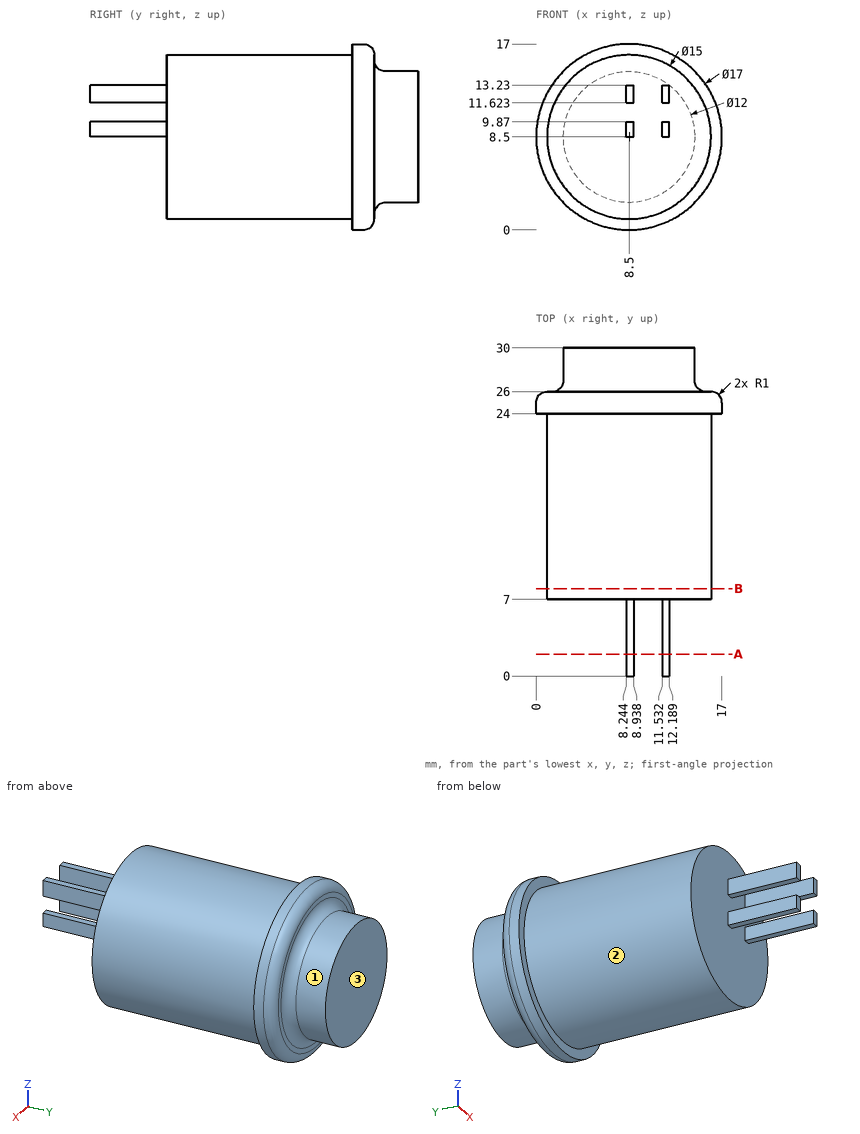
Geometry check sheet. Reference: drawing and pictorial views, mm from the part's lowest x, y, z. A direction names the side the tool comes from. Coordinates: 2 decimals unless noted, no trailing zeros. Write each loop counter-clockwise with the first axis right and the second up, starting at its lowest first coordinate (ties: lowest second). Pieces come first, ordered by that corner, then holes.
Item 1: Scan lines: probe 1 along X at (y, z) = (3, 9) (1 decimal); probe 2 along Z at (x, y) = (13, 13.5); probe 3 along Y at (x, z) = (7.5, 1). Record each from-to range of solid material in increasing order.
Numbers:
probe 1: x = 8.2 to 8.9, 11.5 to 12.2
probe 2: z = 2.5 to 14.5
probe 3: y = 24 to 26
Item 2: Depth check by flat-ended pin: pin 1 Ø8 at (y, z) = (7.5, 9.5) entering from -X; pin 2 Ø5 at (x, y) = (11, 13) entering from -Z; pin 3 Ø5 at (x, y) = (15, 18) entering from -Z (1 decimal). Enter the tip coordinate at first touch or a pass-through.
Numbers:
pin 1: stops at x = 1
pin 2: stops at z = 1
pin 3: stops at z = 2.2
Item 3: Access from +Z, -Z, +X, -X, +Y, -Y to the whole of each face (thin tool, end or side, straight path). Record for the marked faces 1, 2 and 3.
Numbers:
face 1: +Y
face 2: -Y
face 3: +Z, -Z, +X, -X, +Y
Item 4: Cross-section at A-A on y = 2. Record the boundary of the cut face in (x, z) (1 decimal).
Numbers:
outline: (8.2, 8.5) - (8.9, 8.5) - (8.9, 9.9) - (8.2, 9.9) - close; (8.2, 11.6) - (8.9, 11.6) - (8.9, 13.2) - (8.2, 13.2) - close; (11.5, 8.5) - (12.2, 8.5) - (12.2, 9.9) - (11.5, 9.9) - close; (11.5, 11.6) - (12.2, 11.6) - (12.2, 13.2) - (11.5, 13.2) - close
Item 5: Cross-section at B-B on y = 8. Record the boundary of the cut face in (x, z), then the cut area to 3 significant figures.
Numbers:
outline: circle Ø15 at (8.5, 8.5)
area: 177 mm2
